The listing builds one solid part. Answer for the finished solid, in the listing's coordinates (mm). Give positions to 0.01 mm unless a question says otherwise; leave off trailing zeros. Loops run counter-clockwise (first coordinate to the right, second up) from the corner with the lowest first, then second, coordinate; pieces in that order, holes last. Notation, with made-up numbers: (78, -19.5) - (124, -19.5) arc R19 cw to (124, 15.5) - close; hole circle Ø2 at (38, -17.75). An arc over 180 degrees is marked (long way). Write item = value, one per line. Start each with the question number.
1) The part is cut by section B-B on z = 14. State how many separate pieces and enclosed holes the cut face has, plus the area to 3 significant figures.
2) Consider probe 1 along X at (y, z) = (208.28, 16.5); probe 2 along Y at (x, z) = (4, 13); probe 3 along X at (y, z) = (240.5, 0). Determine where each line is inside the solid, lowest interval first.
3) Flat-ended cylindrical pins translate along their axes: P1, Ø3, axis at x = 7.18, y = 101.6, coming from the -Z side; P2, Ø3, axis at y = 169, z = -9, coming from the +X side; P3, Ø4, axis at x = 6.94, y = 139.7, coming from the +Z side. Find the tip coordinate at first contact, or state that the pin passes through.
4) The part is cut by section A-A on y = 196. Write down the section's boundary in (x, z).
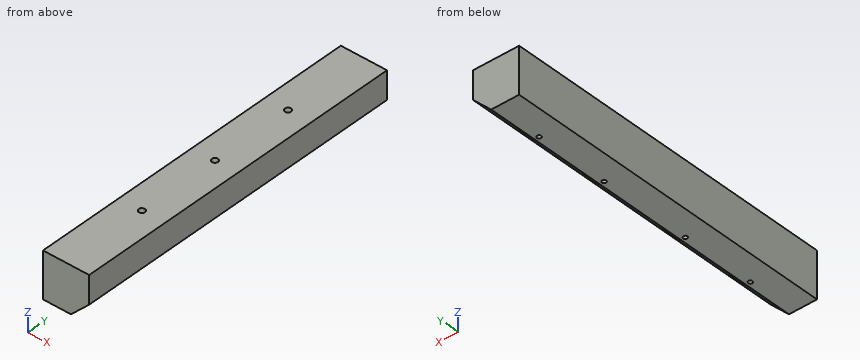
from build123d import *

# Parameters (mm, degrees)
SKETCH1_W                   = 38.1
SKETCH1_H                   = 38.1
BOSS_EXTRUDE1_DEPTH         = 279.4
CHAMFER1_SIZE               = 15
SKETCH15_R                  = 6.35
CUT_EXTRUDE2_DEPTH          = 25
F_1_4_20_TAPPED_HOLE1_D     = 5.1054
F_1_4_20_TAPPED_HOLE1_DEPTH = 20.32
F_1_4_20_TAPPED_HOLE1_TIP   = 1.533816902
F_8_32_TAPPED_HOLE1_REACH   = 285.181
F_8_32_TAPPED_HOLE1_BORE_R  = 1.7272


with BuildPart() as part:
    # Sketch1 → Boss-Extrude1 (new body)
    with BuildSketch(Plane(origin=(0, 0, 0), x_dir=(1, 0, 0), z_dir=(0, 1, 0))):
        with Locations((6.939567467, -5.95)):
            Rectangle(SKETCH1_W, SKETCH1_H)
    extrude(amount=BOSS_EXTRUDE1_DEPTH)

    # Chamfer1
    chamfer1_edges = [part.edges().sort_by_distance(p)[0] for p in [
        (25.989567467, 139.7, -13.1),
    ]]
    chamfer(chamfer1_edges, length=CHAMFER1_SIZE)

    # Sketch15 → Cut-Extrude2 (cut)
    with BuildSketch(Plane(origin=(12.044783734, 0, -12.044783734), x_dir=(-0.7071067811865465, 0, -0.7071067811865487), z_dir=(0.7071067811865487, 0, -0.7071067811865465))):
        with Locations((-9.114300563, 238.76)):
            Circle(SKETCH15_R)
        with Locations((-9.114300563, 177.8)):
            Circle(SKETCH15_R)
        with Locations((-9.114300563, 101.6)):
            Circle(SKETCH15_R)
        with Locations((-9.114300563, 40.64)):
            Circle(SKETCH15_R)
    extrude(amount=-CUT_EXTRUDE2_DEPTH, mode=Mode.SUBTRACT)

    # 1/4-20 Tapped Hole1
    with Locations(Plane.XY.offset(25)):
        with Locations((6.939567467, 208.28), (6.939567467, 139.7), (6.939567467, 71.12)):
            Hole(F_1_4_20_TAPPED_HOLE1_D / 2, depth=F_1_4_20_TAPPED_HOLE1_DEPTH)
            with Locations((0, 0, -(F_1_4_20_TAPPED_HOLE1_DEPTH + F_1_4_20_TAPPED_HOLE1_TIP / 2))):  # 118° drill point
                Cone(0, F_1_4_20_TAPPED_HOLE1_D / 2, F_1_4_20_TAPPED_HOLE1_TIP, mode=Mode.SUBTRACT)

    # #8-32 Tapped Hole1 bore → #8-32 Tapped Hole1 (cut, up to next)
    with BuildSketch(Plane(origin=(0, 0, -13.1), x_dir=(-1, 0, 0), z_dir=(0, 0, -1)), mode=Mode.PRIVATE) as f_8_32_tapped_hole1_sk1:
        with Locations((-7.179567467, 40.64)):
            Circle(F_8_32_TAPPED_HOLE1_BORE_R)
    f_8_32_tapped_hole1_tool1 = extrude(f_8_32_tapped_hole1_sk1.sketch, amount=-F_8_32_TAPPED_HOLE1_REACH, mode=Mode.PRIVATE) & part.part
    # #8-32 Tapped Hole1 bore → #8-32 Tapped Hole1 (cut, up to next)
    with BuildSketch(Plane(origin=(0, 0, -13.1), x_dir=(-1, 0, 0), z_dir=(0, 0, -1)), mode=Mode.PRIVATE) as f_8_32_tapped_hole1_sk2:
        with Locations((-7.179567467, 101.6)):
            Circle(F_8_32_TAPPED_HOLE1_BORE_R)
    f_8_32_tapped_hole1_tool2 = extrude(f_8_32_tapped_hole1_sk2.sketch, amount=-F_8_32_TAPPED_HOLE1_REACH, mode=Mode.PRIVATE) & part.part
    # #8-32 Tapped Hole1 bore → #8-32 Tapped Hole1 (cut, up to next)
    with BuildSketch(Plane(origin=(0, 0, -13.1), x_dir=(-1, 0, 0), z_dir=(0, 0, -1)), mode=Mode.PRIVATE) as f_8_32_tapped_hole1_sk3:
        with Locations((-7.179567467, 177.8)):
            Circle(F_8_32_TAPPED_HOLE1_BORE_R)
    f_8_32_tapped_hole1_tool3 = extrude(f_8_32_tapped_hole1_sk3.sketch, amount=-F_8_32_TAPPED_HOLE1_REACH, mode=Mode.PRIVATE) & part.part
    # #8-32 Tapped Hole1 bore → #8-32 Tapped Hole1 (cut, up to next)
    with BuildSketch(Plane(origin=(0, 0, -13.1), x_dir=(-1, 0, 0), z_dir=(0, 0, -1)), mode=Mode.PRIVATE) as f_8_32_tapped_hole1_sk4:
        with Locations((-7.179567467, 238.76)):
            Circle(F_8_32_TAPPED_HOLE1_BORE_R)
    f_8_32_tapped_hole1_tool4 = extrude(f_8_32_tapped_hole1_sk4.sketch, amount=-F_8_32_TAPPED_HOLE1_REACH, mode=Mode.PRIVATE) & part.part
    add(f_8_32_tapped_hole1_tool1.solids().sort_by_distance((7.179567, 40.64, -13.1))[0], mode=Mode.SUBTRACT)
    add(f_8_32_tapped_hole1_tool2.solids().sort_by_distance((7.179567, 101.6, -13.1))[0], mode=Mode.SUBTRACT)
    add(f_8_32_tapped_hole1_tool3.solids().sort_by_distance((7.179567, 177.8, -13.1))[0], mode=Mode.SUBTRACT)
    add(f_8_32_tapped_hole1_tool4.solids().sort_by_distance((7.179567, 238.76, -13.1))[0], mode=Mode.SUBTRACT)


solid = part.part
Answer below:
q1.separate_pieces = 1
q1.enclosed_holes = 7
q1.area = 10,400 mm2
q2.probe_1 = -12.11 to 4.39, 9.49 to 25.99
q2.probe_2 = 0 to 34.99, 46.29 to 95.95, 107.25 to 172.15, 183.45 to 233.11, 244.41 to 279.4
q2.probe_3 = -12.11 to 4.25, 21.53 to 24.09
q3.P1 = 13.19
q3.P2 = 16.59
q3.P3 = 4.35
q4.outline = (-12.11, -13.1) - (10.99, -13.1) - (25.99, 1.9) - (25.99, 25) - (-12.11, 25) - close
